from build123d import *

# Parameters (mm, degrees)
SKETCH1_W           = 99
SKETCH1_H           = 99
BOSS_EXTRUDE1_DEPTH = 0.5
CUT_EXTRUDE1_DEPTH  = 71.010713466
M2_HOLE1_B_D        = 2.4
M2_HOLE1_B_DEPTH    = 3
M2_HOLE1_B_TIP      = 0.721032743


with BuildPart() as part:
    # Sketch1 → Boss-Extrude1 (new, symmetric)
    with BuildSketch(Plane.XY):
        Rectangle(SKETCH1_W, SKETCH1_H)
    extrude(amount=BOSS_EXTRUDE1_DEPTH, both=True)

    # Sketch2 → Cut-Extrude1 (cut, through all)
    with BuildSketch(Plane.XY.offset(0.5)):
        with BuildLine():
            Line((-49.5, 49.5), (-41, 49.5))
            Line((-41, 49.5), (-41, 42.5))
            ThreePointArc((-41, 42.5), (-41.439339828, 41.439339828), (-42.5, 41))
            Line((-42.5, 41), (-49.5, 41))
            Line((-49.5, 41), (-49.5, 49.5))
        make_face()
        with BuildLine():
            Line((49.5, 49.5), (41, 49.5))
            Line((41, 49.5), (41, 42.5))
            ThreePointArc((41, 42.5), (41.439339828, 41.439339828), (42.5, 41))
            Line((42.5, 41), (49.5, 41))
            Line((49.5, 41), (49.5, 49.5))
        make_face()
        with BuildLine():
            Line((-49.5, -49.5), (-41, -49.5))
            Line((-41, -49.5), (-41, -42.5))
            ThreePointArc((-41, -42.5), (-41.439339828, -41.439339828), (-42.5, -41))
            Line((-42.5, -41), (-49.5, -41))
            Line((-49.5, -41), (-49.5, -49.5))
        make_face()
        with BuildLine():
            Line((49.5, -49.5), (41, -49.5))
            Line((41, -49.5), (41, -42.5))
            ThreePointArc((41, -42.5), (41.439339828, -41.439339828), (42.5, -41))
            Line((42.5, -41), (49.5, -41))
            Line((49.5, -41), (49.5, -49.5))
        make_face()
    extrude(amount=-CUT_EXTRUDE1_DEPTH, mode=Mode.SUBTRACT)

    # M2 Hole1 - B
    with Locations(Plane.XY.offset(0.5)):
        with Locations((-45.75, 29), (-29, 45.75), (29, 45.75), (45.75, 29), (45.75, -29), (29, -45.75), (-29, -45.75), (-45.75, -29)):
            Hole(M2_HOLE1_B_D / 2, depth=M2_HOLE1_B_DEPTH)
            with Locations((0, 0, -(M2_HOLE1_B_DEPTH + M2_HOLE1_B_TIP / 2))):  # 118° drill point
                Cone(0, M2_HOLE1_B_D / 2, M2_HOLE1_B_TIP, mode=Mode.SUBTRACT)


solid = part.part
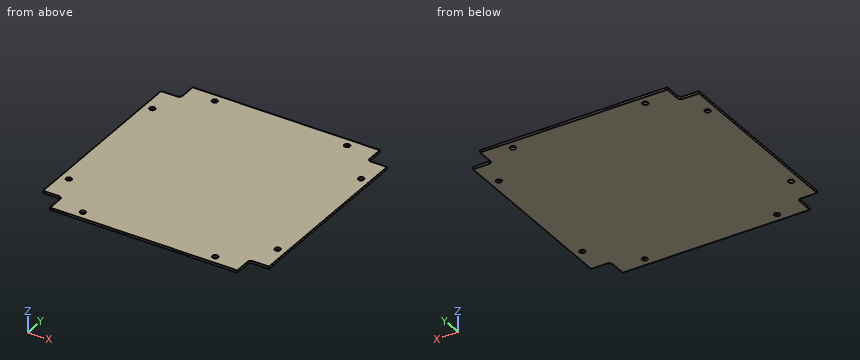
Geometry check sheet. Reference: the model listing, model coordinates, mm. Give positions to 0.01 mm unless a question says otherwise; leave off trailing zeros. Loops run counter-clockwise (first coordinate to the right, second up) from the corner with the lowest first, then second, coordinate; pieces in that order, holes last.
(1) Thickness scan on L1, parallel to Y at x = 29, z = 0.25; L2, parallel to Y at x = 45.75, z = -0.05; L3, parallel to Y at x = -43, z = 0. Record the ranges inside material, lowest first.
From the geometry:
L1: y = -49.5 to -46.95, -44.55 to 44.55, 46.95 to 49.5
L2: y = -41 to -30.2, -27.8 to 27.8, 30.2 to 41
L3: y = -41 to 41
(2) Depth check by flat-ended pin: pin 1 Ø0.5 at (y, z) = (46.5, 0) entering from +X; pin 2 Ø0.5 at (x, z) = (-46.5, 0) entering from +Y; pin 3 Ø0.5 at (y, z) = (-46.5, 0) entering from -X; pin 4 Ø1.4 at (x, y) = (29, 45.75) entering from +Z. Enter the tip coordinate at first touch or a pass-through.
From the geometry:
pin 1: stops at x = 41
pin 2: stops at y = 41
pin 3: stops at x = -41
pin 4: passes through
(3) Section check A-A on x = 29. Record the cut outline in (y, z), then the cut area to 3 significant figures.
From the geometry:
outline: (-49.5, -0.5) - (-46.95, -0.5) - (-46.95, 0.5) - (-49.5, 0.5) - close; (-44.55, -0.5) - (44.55, -0.5) - (44.55, 0.5) - (-44.55, 0.5) - close; (46.95, -0.5) - (49.5, -0.5) - (49.5, 0.5) - (46.95, 0.5) - close
area: 94.2 mm2
(4) Section check C-C on z = 0.1. Count the separate pieces of the cut face and the enclosed holes in it, then the cut area to 3 significant figures.
From the geometry:
separate pieces: 1
enclosed holes: 8
area: 9,480 mm2
